Check sheet for the modelled part. Datum: model origin and axes. Units: mm. Face numbers are marked on the shaded views. A direction names the side the tool comes from. Coordinates: 2 decimals unless noted, no trailing zeros. Loops run counter-clockwise (first coordinate to the right, second up) from the corner with the lowest first, then second, coordinate; pieces in that order, holes last.
```python
from build123d import *

# Parameters (mm, degrees)
SKETCH_1_W             = 28
SKETCH_1_H             = 160
SKETCH_1_R             = 1.25
SM_BASE_FLANGE_1_DEPTH = 3
OTHER_START            = -14
OTHER_1_DEPTH          = 28
OTHER_1_2_DEPTH        = 28
SKETCH_7_R             = 1.35
CUT_EXTRUDE_1_DEPTH    = 81.582164958


# Read off the part's stored shape, not the designer's step: 绘制的折弯1
# Sheet-metal steps are written as plain solids
with BuildPart() as part:
    # Sketch 1 → 基体-法兰1 (new body)
    with BuildSketch(Plane(origin=(0, 0, 0), x_dir=(1, 0, 0), z_dir=(0, 1, 0))):
        Rectangle(SKETCH_1_W, SKETCH_1_H)
        with Locations(Location((-11, -16, 0), (0, 0, 90))):
            Circle(SKETCH_1_R, mode=Mode.SUBTRACT)
        with Locations(Location((11, -16, 0), (0, 0, 270))):
            Circle(SKETCH_1_R, mode=Mode.SUBTRACT)
        with Locations(Location((11, 16, 0), (0, 0, 90))):
            Circle(SKETCH_1_R, mode=Mode.SUBTRACT)
        with Locations(Location((-11, 16, 0), (0, 0, 270))):
            Circle(SKETCH_1_R, mode=Mode.SUBTRACT)
    extrude(amount=-SM_BASE_FLANGE_1_DEPTH)

    # Other 1 outline → Other 1 (cut)
    with BuildSketch(Plane.YZ.offset(OTHER_START)):
        with BuildLine():
            ThreePointArc((0, -31.146677222), (-2.154295979, -29.850867001), (-3, -27.4834))
            Line((-3, -27.4834), (-3, -80))
            Line((-3, -80), (0, -80))
            Line((0, -80), (0, -31.146677222))
        make_face()
        with BuildLine():
            Line((-3, 80), (-3, 22.7634))
            ThreePointArc((-3, 22.7634), (-2.154295979, 25.130867001), (0, 26.426677222))
            Line((0, 26.426677222), (0, 80))
            Line((0, 80), (-3, 80))
        make_face()
    extrude(amount=OTHER_1_DEPTH, mode=Mode.SUBTRACT)

    # Other 1 2 outline → Other 1 2 (add)
    with BuildSketch(Plane.YZ.offset(OTHER_START)):
        with BuildLine():
            Line((0, -27.4834), (0, -31.146677222))
            ThreePointArc((0, -31.146677222), (0.36647982, -31.201624121), (0.7366, -31.22))
            Line((0.7366, -31.22), (49.739956935, -31.22))
            Line((49.739956935, -31.22), (49.739956935, -28.22))
            Line((49.739956935, -28.22), (0.7366, -28.22))
            ThreePointArc((0.7366, -28.22), (0.215745145, -28.004254855), (0, -27.4834))
        make_face()
        with BuildLine():
            ThreePointArc((0.7366, 26.5), (0.36647982, 26.481624121), (0, 26.426677222))
            Line((0, 26.426677222), (0, 22.7634))
            ThreePointArc((0, 22.7634), (0.215745145, 23.284254855), (0.7366, 23.5))
            Line((0.7366, 23.5), (54.459956935, 23.5))
            Line((54.459956935, 23.5), (54.459956935, 26.5))
            Line((54.459956935, 26.5), (0.7366, 26.5))
        make_face()
    extrude(amount=OTHER_1_2_DEPTH)

    # Sketch 7 → 切除-拉伸1 (cut, through all)
    with BuildSketch(Plane(origin=(0, 0, -31.22), x_dir=(-1, 0, 0), z_dir=(0, 0, -1))):
        with Locations(Location((11, 27, 0), (0, 0, 90))):
            Circle(SKETCH_7_R)
        with Locations(Location((7.778174593, 19.221825407, 0), (0, 0, 90))):
            Circle(SKETCH_7_R)
        with Locations(Location((0, 16, 0), (0, 0, 90))):
            Circle(SKETCH_7_R)
        with Locations(Location((-7.778174593, 19.221825407, 0), (0, 0, 90))):
            Circle(SKETCH_7_R)
        with Locations(Location((-11, 27, 0), (0, 0, 90))):
            Circle(SKETCH_7_R)
        with BuildLine():
            Line((-14, 27), (-32.703539992, 27))
            Line((-32.703539992, 27), (-27.737483214, 57.366036836))
            Line((-27.737483214, 57.366036836), (24.538070134, 57.366036836))
            Line((24.538070134, 57.366036836), (24.538070134, 27))
            Line((24.538070134, 27), (14, 27))
            Line((14, 27), (14, 30))
            Line((14, 30), (6, 30))
            Line((6, 30), (6, 27))
            ThreePointArc((6, 27), (0, 21), (-6, 27))
            Line((-6, 27), (-6, 30))
            Line((-6, 30), (-14, 30))
            Line((-14, 30), (-14, 27))
        make_face()
    extrude(amount=-CUT_EXTRUDE_1_DEPTH, mode=Mode.SUBTRACT)


solid = part.part
```
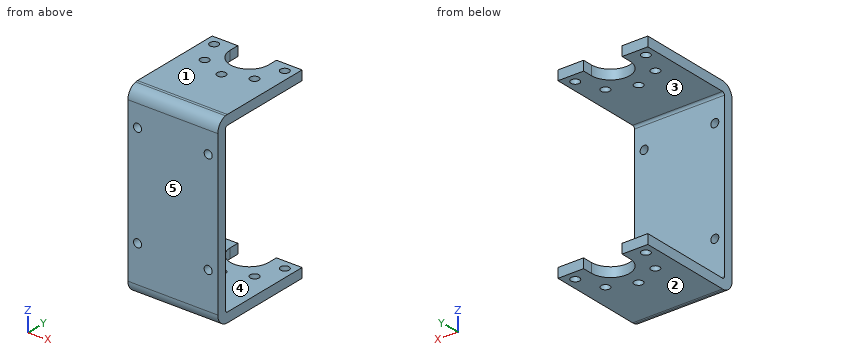
1) Mould release check, pull along Z, two halves, no side actions. Record for the marked faces 1, 2 and 3: +Z half, -Z half, draft (parallel to the pull), parting line (faces both ways), or undercut.
Answer sheet:
face 1: +Z half
face 2: -Z half
face 3: undercut
2) Section check C-C on y = 10. Enter the section's corners in (x, z), plus the area to 3 significant figures.
Answer sheet:
outline: (-14, -31.22) - (14, -31.22) - (14, -28.22) - (-14, -28.22) - close; (-14, 23.5) - (14, 23.5) - (14, 26.5) - (-14, 26.5) - close
area: 168 mm2
3) Depth check by flat-ended pin: pin 1 (1.5 mm diameter, centred on x = -11, z = -20.5, fed in from +Y). Enter the tip coordinate at first touch or a pass-through.
Answer sheet:
pin 1: stops at y = 0
4) Section check B-B on z = 16. Enter the section's corners in (x, y), plus the area to 3 significant figures.
Answer sheet:
outline: (-14, -3) - (-12.25, -3) - (-12.25, 0) - (-14, 0) - close; (-9.75, -3) - (9.75, -3) - (9.75, 0) - (-9.75, 0) - close; (12.25, -3) - (14, -3) - (14, 0) - (12.25, 0) - close
area: 69.0 mm2
5) Section check A-A on y = 16. Enter the section's corners in (x, z).
Answer sheet:
outline: (-14, -31.22) - (-1.35, -31.22) - (-1.35, -28.22) - (-14, -28.22) - close; (-14, 23.5) - (-1.35, 23.5) - (-1.35, 26.5) - (-14, 26.5) - close; (1.35, -31.22) - (14, -31.22) - (14, -28.22) - (1.35, -28.22) - close; (1.35, 23.5) - (14, 23.5) - (14, 26.5) - (1.35, 26.5) - close
6) Scan lines: line 1 (X direction, y = 27, z = 24); line 2 (Z direction, x = -5.25, y = 21.5); line 3 (Y direction, x = -6.5, z = -15.5). Record each from-to range of solid material in increasing order.
Answer sheet:
line 1: x = -14 to -12.35, -9.65 to -6, 6 to 9.65, 12.35 to 14
line 2: z = -31.22 to -28.22, 23.5 to 26.5
line 3: y = -3 to 0
7) Set-up check for the marked faces 4 and 5: record each of +Z, -Z, +X, -X, +Y, -Y from which the full face is reachable in a straight line by a thin tool's end or side.
Answer sheet:
face 4: +X, -X, +Y
face 5: +Z, -Z, +X, -X, -Y
8) Section check D-D on x = 11. Enter the section's corners in (y, z), plus the area to 3 significant figures.
Answer sheet:
outline: (-3, -27.48) arc R3.74 ccw to (0.74, -31.22) - (25.65, -31.22) - (25.65, -28.22) - (0.74, -28.22) arc R0.74 cw to (0, -27.48) - (0, -17.25) - (-3, -17.25) - close; (-3, -14.75) - (0, -14.75) - (0, 14.75) - (-3, 14.75) - close; (-3, 17.25) - (0, 17.25) - (0, 22.76) arc R0.74 cw to (0.74, 23.5) - (25.65, 23.5) - (25.65, 26.5) - (0.74, 26.5) arc R3.74 ccw to (-3, 22.76) - close; (28.35, -31.22) - (30, -31.22) - (30, -28.22) - (28.35, -28.22) - close; (28.35, 23.5) - (30, 23.5) - (30, 26.5) - (28.35, 26.5) - close
area: 316 mm2
